Geometry check sheet. Reference: the model listing, model coordinates, mm. A direction names the side the tool comes from. Give positions to 0.01 mm unless a question says otherwise; leave off trailing zeros. Write each loop counter-clockwise with the first axis right and the second up, starting at its lowest first coordinate (ties: lowest second). Pieces come first, ordered by that corner, then holes. Notation, with made-up numbers: (62, 69.25) - (116, 69.25) arc R26 cw to (116, 86.25) - close; hole circle Ø3 at (58, -8). An arc over 180 degrees is marked (long way). One line per question, with ' | ' between items. Start each with the question number.
Q1. Section check B-B on y = 0. Record the boundary of the cut face in (x, z).
Q2. Section check A-A on z = 47. Record the boundary of the cut face in (x, y).
Q3. Set-up check for faces 1 (the face through (28, 45, 1)), 2 (the face through (20.765, -39.923, 100.386)), 3 (the face through (-4, -47, 2)): record each of +Z, -Z, +X, -X, +Y, -Y from which the full face is reachable in a straight line by a thin tool's end or side.
Q4. Thickness scan on L1, parallel to Y at x = 0, z = 110; L2, parallel to Z at x = -19.5, y = 44; L3, parallel to Z at x = 31.5, y = 5. Record the ranges inside material, lowest first. Write a range as [from, to].
Q5. Gauge pin test, flat ends, axial feed: P1, Ø12, axis at x = 11.5, z = 128, coming from the +Y side; P2, Ø3, axis at x = 20.5, z = 103.5, coming from the +Y side; P3, Ø10, axis at y = -13, z = 172.5, coming from the -X side. Record the tip position at first contact, or that the pin passes through.
Q6. Release check for a two-part mould opening along Y. For faces 4 (the face through (-1, 1, 198)), 5 (the face through (-24, -39, 0)), 6 (the face through (44.83, 14.12, 99.61)) record: +Y half, -Y half, draft (parallel to the pull), parting line (faces both ways), or undercut.
```python
from build123d import *

# Parameters (mm, degrees)
F0_R     = 53
F0_R_2   = 47
F1_DEPTH = 2
F2_DEPTH = 200
F3_T     = 2


# Not quite as in the source:
# - a shell that OpenCascade refuses in one call is made with other operations: the cavity is built on its own and cut out


with BuildPart() as f1:
    # F0 (on Top) → F1 (new body)
    with BuildSketch(Plane.XY):
        Circle(F0_R)
        Circle(F0_R_2, mode=Mode.SUBTRACT)
    extrude(amount=F1_DEPTH)

    # F0 (on Top) → F2 (join)
    with BuildSketch(Plane.XY):
        Circle(F0_R_2)
    extrude(amount=F2_DEPTH)

    # F3: shell of thickness 2, made by hand


with BuildPart() as f3_core1:
    # F3_t2: copy of F1
    add(f1.part)

    # the walls: a layer under each face that stays
    f3_faces = [f3_core1.faces().sort_by_distance(p)[0] for p in [
        (-53, 0, 1),
        (-35.3333333333, -35.3333333333, 2),
        (-47, 0, 101),
        (0, 0, 200),
    ]]
    thicken(f3_faces, amount=-F3_T, mode=Mode.SUBTRACT)

    # F3_s3 → F3_t4 (revolve, cut)
    with BuildSketch(Plane.XZ):
        Polygon((47.02, 2.02), (47, 0), (45, 0), (45, 2), align=None)
    revolve(axis=Axis((0, 0, 2), (0, 0, 1)), mode=Mode.SUBTRACT)


with BuildPart() as f1_1:
    add(f1.part)

    # what is left inside the walls is the cavity
    f3_cavity = [f3_core1.part.solids().sort_by_distance(p)[0] for p in [
        (-44.98, 0, 132.666667),
    ]]
    add(f3_cavity, mode=Mode.SUBTRACT)


solid = f1_1.part
```
Working result:
1) outline: (-53, 0) - (-45, 0) - (-45, 198) - (45, 198) - (45, 0) - (53, 0) - (53, 2) - (47, 2) - (47, 200) - (-47, 200) - (-47, 2) - (-53, 2) - close
2) outline: circle Ø94 at (0, 0); hole circle Ø90 at (0, 0)
3) face 1: +Z, -Z | face 2: -Z | face 3: +Z
4) L1: y = [-47, -45], [45, 47] | L2: z = [0, 2] | L3: z = [198, 200]
5) P1: stops at y = 46.68 | P2: stops at y = 42.99 | P3: stops at x = -46.31
6) face 4: undercut | face 5: draft | face 6: parting line
